Here's how the part is built. I have some questions about the finished solid (model axes, mm). Face numbers are marked on the shaded views. A direction names the side the tool comes from. Give positions to 0.01 mm unless a question says otherwise; leave off trailing zeros. Loops run counter-clockwise (first coordinate to the right, second up) from the corner with the lowest first, then second, coordinate; pieces in that order, holes last.
Q1. For the marked faces 4, 5, 6, 7 and 8, which set-ups out of +Z, -Z, +X, -X, +Y, -Y let a thin tool reach every point of the face, with its end or its side?
Q2. We'd pull the mould along X, two halves only. Please class the marked faces 1, 2 and 3: +X half, -X half, draft (parallel to the pull), parting line (faces both ways), or undercut.
Q3. I need wall thicknesses on line 1 (X direction, y = -11.75, z = -97.5); line 2 (Z direction, x = -0.5, y = -1.5); line 3 (X direction, y = -15, z = -105). Which ranges of each line are inside material? Lowest first, please.
Q4. If we section it at A-A (z = 81): Please give me the cut outline in (x, y), plus the area to 3 significant figures.
Q5. Will these pins go through, and if not, where does the flat tip stop? P1, Ø5, axis at x = 18, z = -12.5, coming from the +Y side; P2, Ø6, axis at y = -11, z = 7, coming from the +X side; P3, Ø1.5, axis at x = -66.5, y = -9.5, coming from the +Z side; P4, Ø8, axis at x = -95.5, z = -2, coming from the +Y side.
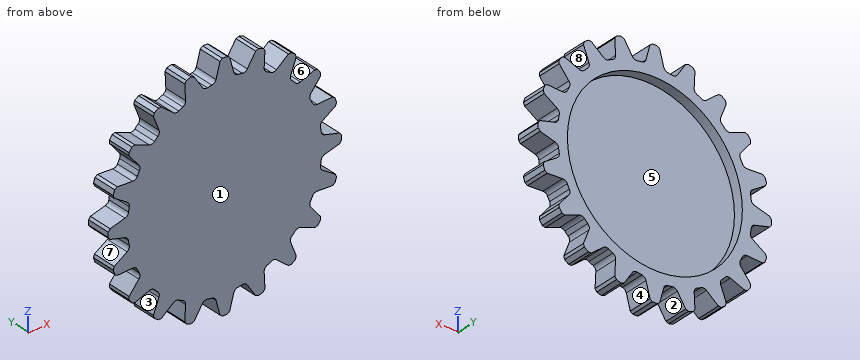
from build123d import *

# Parameters (mm, degrees)
F0_R            = 100
F1_DEPTH        = 25
F3_DEPTH        = 25
F3_COPIES_COUNT = 20
F4_SIZE         = 2
F5_R            = 5
F6_R            = 90
F7_DEPTH        = 10


# Not quite as in the source:
# - a pattern or mirror of a feature is missing from the dataset's text; its kind, count and spacing are read off the source's solid


with BuildPart() as f1:
    # F0 (on Front) → F1 (new body)
    with BuildSketch(Plane.XZ):
        Circle(F0_R)
    extrude(amount=F1_DEPTH)

    # F2 (on Front) → F3 (join)
    with BuildSketch(Plane.XZ):
        Polygon((-4.5, 120), (-9.9931095726, 99.4994359837), (9.9931095726, 99.4994359837), (4.5, 120), align=None)
    f3 = extrude(amount=F3_DEPTH)

    # F3_copies: F3 ×20 about axis
    f3_copies_axis = Axis((0, 0, 0), (0, 1, 0))
    for i in range(1, F3_COPIES_COUNT):
        add(f3.rotate(f3_copies_axis, i * 360 / F3_COPIES_COUNT))

    # F4
    f4_edges = [f1.edges().sort_by_distance(p)[0] for p in [
        (-4.5, -12.5, 120),
        (4.5, -12.5, 120),
        (-32.802285, -12.5, 115.517358),
        (115.517358, -12.5, 32.802285),
        (120, -12.5, 4.5),
        (120, -12.5, -4.5),
        (115.517358, -12.5, -32.802285),
        (112.736205, -12.5, -41.361794),
        (99.727073, -12.5, -66.893654),
        (94.437006, -12.5, -74.174807),
        (74.174807, -12.5, -94.437006),
        (66.893654, -12.5, -99.727073),
        (41.361794, -12.5, -112.736205),
        (32.802285, -12.5, -115.517358),
        (4.5, -12.5, -120),
        (-4.5, -12.5, -120),
        (-32.802285, -12.5, -115.517358),
        (-41.361794, -12.5, -112.736205),
        (-66.893654, -12.5, -99.727073),
        (-74.174807, -12.5, -94.437006),
        (-94.437006, -12.5, -74.174807),
        (-99.727073, -12.5, -66.893654),
        (-112.736205, -12.5, -41.361794),
        (-115.517358, -12.5, -32.802285),
        (-120, -12.5, -4.5),
        (-120, -12.5, 4.5),
        (-115.517358, -12.5, 32.802285),
        (-112.736205, -12.5, 41.361794),
        (-99.727073, -12.5, 66.893654),
        (-94.437006, -12.5, 74.174807),
        (-74.174807, -12.5, 94.437006),
        (-66.893654, -12.5, 99.727073),
        (32.802285, -12.5, 115.517358),
        (41.361794, -12.5, 112.736205),
        (66.893654, -12.5, 99.727073),
        (74.174807, -12.5, 94.437006),
        (94.437006, -12.5, 74.174807),
        (99.727073, -12.5, 66.893654),
        (112.736205, -12.5, 41.361794),
        (-41.361794, -12.5, 112.736205),
    ]]
    chamfer(f4_edges, length=F4_SIZE)

    # F5
    f5_edges = [f1.edges().sort_by_distance(p)[0] for p in [
        (-9.99311, -12.5, 99.499436),
        (9.99311, -12.5, 99.499436),
        (97.717628, -12.5, 21.243005),
        (99.499436, -12.5, 9.99311),
        (91.541546, -12.5, 40.251029),
        (86.370537, -12.5, 50.399706),
        (99.499436, -12.5, -9.99311),
        (97.717628, -12.5, -21.243005),
        (74.622932, -12.5, 66.568897),
        (66.568897, -12.5, 74.622932),
        (91.541546, -12.5, -40.251029),
        (86.370537, -12.5, -50.399706),
        (50.399706, -12.5, 86.370537),
        (40.251029, -12.5, 91.541546),
        (74.622932, -12.5, -66.568897),
        (66.568897, -12.5, -74.622932),
        (21.243005, -12.5, 97.717628),
        (50.399706, -12.5, -86.370537),
        (40.251029, -12.5, -91.541546),
        (-21.243005, -12.5, 97.717628),
        (21.243005, -12.5, -97.717628),
        (9.99311, -12.5, -99.499436),
        (-40.251029, -12.5, 91.541546),
        (-50.399706, -12.5, 86.370537),
        (-9.99311, -12.5, -99.499436),
        (-21.243005, -12.5, -97.717628),
        (-66.568897, -12.5, 74.622932),
        (-74.622932, -12.5, 66.568897),
        (-40.251029, -12.5, -91.541546),
        (-50.399706, -12.5, -86.370537),
        (-86.370537, -12.5, 50.399706),
        (-91.541546, -12.5, 40.251029),
        (-66.568897, -12.5, -74.622932),
        (-74.622932, -12.5, -66.568897),
        (-97.717628, -12.5, 21.243005),
        (-99.499436, -12.5, 9.99311),
        (-86.370537, -12.5, -50.399706),
        (-91.541546, -12.5, -40.251029),
        (-99.499436, -12.5, -9.99311),
        (-97.717628, -12.5, -21.243005),
    ]]
    fillet(f5_edges, radius=F5_R)

    # F6 (on face) → F7 (cut)
    with BuildSketch(Plane(origin=(0, 0, 0), x_dir=(-1, 0, 0), z_dir=(0, 1, 0))):
        Circle(F6_R)
    extrude(amount=-F7_DEPTH, mode=Mode.SUBTRACT)


solid = f1.part
Check sheet entries:
1. face 4: -Z, +Y, -Y
1. face 5: +Y
1. face 6: +Z, +Y, -Y
1. face 7: -X, +Y, -Y
1. face 8: +X, +Y, -Y
2. face 1: draft
2. face 2: undercut
2. face 3: -X half
3. line 1: x = -69.96 to -64.14, -40.56 to 40.56, 64.14 to 69.96
3. line 2: z = -120 to -90, 90 to 120
3. line 3: x = -40.96 to -25.97, -8.52 to 8.52, 25.97 to 40.96
4. outline: (-69.02, -25) - (69.02, -25) - (69.02, 0) - (39.23, 0) - (39.23, -10) - (-39.23, -10) - (-39.23, 0) - (-69.02, 0) - close
4. area: 2,670 mm2
5. P1: stops at y = -10
5. P2: stops at x = 118.85
5. P3: stops at z = 98.52
5. P4: stops at y = 0
